Here's how the part is built. I have some questions about the finished solid (model axes, mm). Face numbers are marked on the shaded views. A direction names the side the tool comes from. Round coordinates to 2 decimals unless told otherwise and drop trailing zeros. Write each loop counter-clockwise with the first axis right and the second up, starting at its lowest first coordinate (ties: lowest second). Pieces come first, ordered by that corner, then holes. Notation, with made-up numbers: M 49.5,25.5 L 60.5,25.5 A18 cw 60.5,51.5 Z; hole C 83,-37.5 d8. An arc over 180 degrees is marked long. Use a Markdown table: item, result. Add a question column.
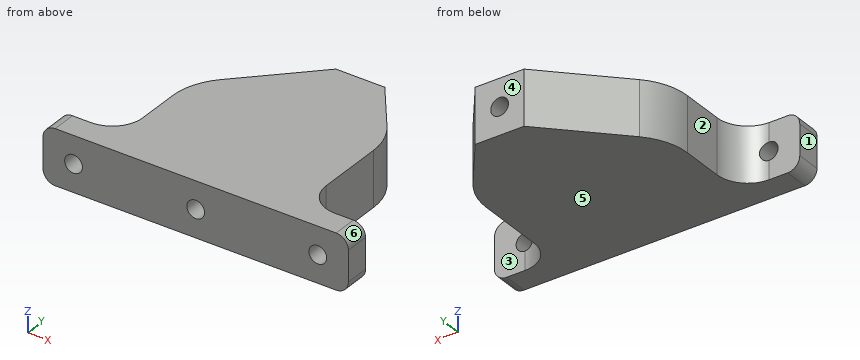
Autodesk Inventor part; units mm, degrees
ref_plane "YZ Plane" through (0, 0, 0) normal (1, 0, 0) x (0, 1, 0)
ref_plane "XZ Plane" through (0, 0, 0) normal (0, 1, 0) x (-1, 0, 0)
ref_plane "XY Plane" through (0, 0, 0) normal (0, 0, 1) x (1, 0, 0)
sketch "Sketch1" plane through (0, 0, 0) normal (0, 0, 1) x (1, 0, 0)
  line L0 (-25, -5) -> (25, -5)
  line L1 (25, -5) -> (25, 5)
  line L2 (25, 5) -> (-25, 5)
  line L3 (-25, 5) -> (-25, -5)
  line L4 (-25, -5) -> (25, 5) construction
  line L5 (25, -5) -> (-25, 5) construction
  line L6 (-25, 5) -> (-1, 29)
  line L7 (-1, 29) -> (7, 29)
  line L8 (7, 29) -> (25, 5)
  line L9 (3, 29) -> (3, 5) construction
  point P0 (0, 0)
  dimension "d0" = 28
  dimension "d1" = 50
  dimension "d2" = 34
  dimension "d3" = 8
  dimension "d4" = 10
extrude "Extrusion1" add sketch "Sketch1" along normal blind 9
sketch "Sketch2" plane through (-25, -5, 0) normal (0, -1, 0) x (1, 0, 0)
  line L0 (0, 0) -> (50, 0)
  line L1 (50, 0) -> (50, 9)
  line L2 (0, 9) -> (50, 9)
  line L3 (0, 0) -> (0, 9)
  point P0 (25, 0)
  point P1 (5, 4.5)
  point P2 (25, 4.5)
  point P3 (45, 4.5)
  point P4 (50, 4.5)
  dimension "d7" = 20
  dimension "d8" = 20
  dimension "d9" = 5
hole "Hole1" at (20, -5, 4.5) at (-20, -5, 4.5) at (0, -5, 4.5) direction (0, 1, 0) diameter 2.9 depth 10
sketch "Sketch3" plane through (-1, 29, 0) normal (0, 1, 0) x (1, 0, 0)
  line L0 (8, 0) -> (0, 0)
  line L1 (0, 0) -> (0, -9)
  line L2 (8, -9) -> (0, -9)
  line L3 (8, 0) -> (8, -9)
  point P0 (1, 0)
  point P1 (4, -4.5)
  point P2 (8, -4.5)
  point P3 (4, 0)
hole "Hole2" at (3, 29, 4.5) direction (0, -1, 0) diameter 2.9 depth 20
sketch "Sketch4" plane through (0, 0, 0) normal (0, 0, -1) x (-1, 0, 0)
  line L0 (-18.55, -5) -> (-21.45, -5)
  line L1 (-21.45, 5) -> (-18.55, 5)
  line L2 (-25, -5) -> (-25, 5)
  line L3 (-25, -1) -> (-15, -1)
  line L4 (-15, -1) -> (-15, 18.3333)
  line L5 (25, -5) -> (-25, -5)
  line L6 (-7, 29) -> (1, 29)
  line L7 (-25, 5) -> (-7, 29)
  line L8 (-25, -5) -> (-25, 5)
  line L9 (25, -5) -> (-25, -5)
  line L10 (25, 5) -> (25, -5)
  line L11 (1, 29) -> (25, 5)
  line L12 (21.45, 5) -> (21.45, -5)
  line L13 (18.55, 5) -> (18.55, -5)
  line L14 (-15, -1) -> (25, -1)
  line L15 (15, -1) -> (15, 15)
  point P0 (0, 0)
  dimension "d25" = 3.55
  dimension "d26" = 4
  dimension "d27" = 3.55
extrude "Extrusion2" cut sketch "Sketch4" against normal through all contours L14 L15 L11 L10 | L2 L7 L4 L3
fillet "Fillet2" radius 5 2 edges at (15, -1, 4.5) (-15, -1, 4.5)
fillet "Fillet3" radius 2 4 edges at (25, -3, 0) (25, -3, 9) (-25, -3, 0) (-25, -3, 9)
fillet "Fillet4" radius 10 2 edges at (-15, 15, 4.5) (15, 18.3333, 4.5)
equation "\"d27\" = d25"
properties part number "LeftLevelBlock" material "ABS Plastic"
Item 1: For pin 1 Ø4 at (y, z) = (13, 6) entering from +X; pin 2 Ø1.5 at (x, z) = (-22, 5.5) entering from +Y; pin 3 Ø3.5 at (y, z) = (6, 6.5) entering from -X, each with a flat end and sliding along its axis, tell me the tip position at first contact or that it passes through.
Item 2: If we mould it in two halves opening along Z, with no side actions, what happens to the marked faces 4, 5 and 6? For each: +Z half, -Z half, draft (parallel to the pull), parting line (faces both ways), or undercut.
Item 3: Imagine slicing it at C-C on y = 21.5. List the corners of the cut face in (x, z) for me (3 decimals).
Item 4: On a 3-axis mill with a long thin cutter (end or side, diameter ignored), from which of +Z, -Z, +X, -X, +Y, -Y can I reach the whole of each face in a straight line? I mean the marked faces 1, 2 and 3. Say none if no direction works.
Item 5: Imagine slicing it at B-B on x = 3. List the corners of the cut face in (y, z) for me.
Item 6: Imagine slicing it at A-A on z = 4.5. List the corners of the cut face in (x, y) for me, plus the area to 3 significant figures.
Item 7: Imagine slicing it at D-D on z = 0.5. List the corners of the cut face in (x, y) for me, plus the area to 3 significant figures.
Item 8: I need wall thicknesses on probe 1 along X at (y, z) = (-3.5, 4.5); probe 2 along Z at (x, y) = (20, -2.75); probe 3 along X at (y, z) = (7.5, 0.5). Which ranges of each line are inside material? Lowest first, please. Write a range as from..to.
The answers:
| question | item | result |
|---|---|---|
| 1 | pin 1 | x = 15 |
| 1 | pin 2 | y = -1 |
| 1 | pin 3 | x = -15 |
| 2 | face 4 | draft |
| 2 | face 5 | -Z half |
| 2 | face 6 | +Z half |
| 3 | outline | M -8.5,0 L 12.625,0 L 12.625,9 L -8.5,9 Z; hole C 3,4.5 d2.9 |
| 4 | face 1 | +Z, -Z, -X, +Y, -Y |
| 4 | face 2 | +Z, -Z, -X, +Y |
| 4 | face 3 | +Z, -Z, +X, +Y |
| 5 | outline | M -5,0 L 29,0 L 29,3.05 L 9,3.05 L 9,5.95 L 29,5.95 L 29,9 L -5,9 Z |
| 6 | outline | M -25,-5 L -21.45,-5 L -21.45,-1 L -25,-1 Z; M -18.55,-5 L -1.45,-5 L -1.45,5 L 1.45,5 L 1.45,-5 L 18.55,-5 L 18.55,-0.79 A5 cw 15,4 L 15,15 A10 ccw 13,21 L 7,29 L 4.45,29 L 4.45,9 L 1.55,9 L 1.55,29 L -1,29 L -12.07,17.93 A10 ccw -15,10.86 L -15,4 A5 cw -18.55,-0.79 Z; M 21.45,-5 L 25,-5 L 25,-1 L 21.45,-1 Z |
| 6 | area | 856 mm² |
| 7 | outline | M -24.32,-5 L 24.32,-5 L 24.32,-1 L 20,-1 A5 cw 15,4 L 15,15 A10 ccw 13,21 L 7,29 L -1,29 L -12.07,17.93 A10 ccw -15,10.86 L -15,4 A5 cw -20,-1 L -24.32,-1 Z |
| 7 | area | 961 mm² |
| 8 | probe 1 | -25..-21.45, -18.55..-1.45, 1.45..18.55, 21.45..25 |
| 8 | probe 2 | 0..3.05, 5.95..9 |
| 8 | probe 3 | -15..15 |
